Here's how the part is built. I have some questions about the finished solid (model axes, mm). Face numbers are marked on the shaded views. A direction names the side the tool comes from. Round coordinates to 2 decimals unless told otherwise and drop trailing zeros. Write each loop counter-clockwise with the first axis right and the second up, starting at its lowest first coordinate (ties: lowest second). Pieces come first, ordered by that corner, then holes. Notation, with made-up numbers: (10.25, 39.25) - (24.25, 39.25) arc R14 cw to (24.25, 65.25) - close; hole circle Ø2 at (-1.5, 63.25). An arc over 180 degrees is marked (long way). Write item = value, one per line. Start each with the question number.
Item 1: If we section it at A-A (x = 12): Please give me the cut outline in (y, z).
Item 2: If we section it at B-B (y = -110.5): Give the number of separate pieces and of enclosed holes in the cut face, and give its area (3 significant figures).
Item 3: If I drill on line 1 along Z through (x, y) = (9, 0); line 2 along Y through (x, z) = (3.5, -13); line 3 along X through (y, z) = (127, -56.5), over which ranges is the centre line in solid material (lowest first)? Write a range as [from, to].
Item 4: Which directions (+Z, -Z, +X, -X, +Y, -Y) give clear straight access to the entire face, cutting with the end or side of a thin tool? Please do the marked faces 1 and 2.
Item 5: For P1, Ø6, axis at x = 0, y = -110.5, coming from the +Z side; P2, Ø12, axis at y = -100.5, z = 28, coming from the +X side; P3, Ø1.8, axis at x = -1, z = 79, coming from the +Y side, each with a flat end and sliding along its axis, tell me the tip position at first contact or that it passes through.
```python
from build123d import *

# Parameters (mm, degrees)
F0_R          = 150
F0_R_2        = 137.5
F1_DEPTH      = 8
F1_DEPTH_BACK = 8
F0_R_3        = 15
F2_DEPTH      = 3
F2_DEPTH_BACK = 3
F0_R_4        = 11
F3_DEPTH      = 25
F3_DEPTH_BACK = 5
F4_R          = 4


with BuildPart() as f1:
    # F0 (on Right) → F1 (new body, two sides)
    with BuildSketch(Plane.YZ) as f1_sk:
        Circle(F0_R)
        with Locations((2.112069, 0)):
            Circle(F0_R_2, mode=Mode.SUBTRACT)
    extrude(amount=F1_DEPTH)
    extrude(f1_sk.sketch, amount=-F1_DEPTH_BACK)

    # F0 (on Right) → F2 (join, two sides)
    with BuildSketch(Plane.YZ) as f2_sk:
        with Locations((2.112069, 0)):
            Circle(F0_R_2)
        with BuildLine():
            ThreePointArc((-20.96825, -1.5987), (-18.909393, -2.888208), (-17.701314, -4.995877))
            ThreePointArc((-17.701314, -4.995877), (-17.492598, -5.68369), (-17.257166, -6.362822))
            ThreePointArc((-17.257166, -6.362822), (-16.995666, -8.778053), (-17.903363, -11.031452))
            Line((-17.903363, -11.031452), (-80.155489, -96.714153))
            ThreePointArc((-80.155489, -96.714153), (-83.705152, -98.750622), (-87.586694, -97.454111))
            ThreePointArc((-87.586694, -97.454111), (-124.025507, -40.404007), (-127.515568, 27.200141))
            ThreePointArc((-127.515568, 27.200141), (-125.127779, 30.500202), (-121.077051, 30.928621))
            Line((-121.077051, 30.928621), (-20.96825, -1.5987))
        make_face(mode=Mode.SUBTRACT)
        with BuildLine():
            ThreePointArc((67.077994, -115.42357), (0.327024, -132.43861), (-65.941115, -113.6307))
            ThreePointArc((-65.941115, -113.6307), (-68.271016, -110.341527), (-67.417198, -106.402225))
            Line((-67.417198, -106.402225), (-4.959091, -20.436016))
            ThreePointArc((-4.959091, -20.436016), (-3.096475, -18.876406), (-0.718646, -18.378761))
            ThreePointArc((-0.718646, -18.378761), (0, -18.392806), (0.718646, -18.378761))
            ThreePointArc((0.718646, -18.378761), (3.096475, -18.876406), (4.959091, -20.436016))
            Line((4.959091, -20.436016), (68.670621, -108.127414))
            ThreePointArc((68.670621, -108.127414), (69.510512, -112.132647), (67.077994, -115.42357))
        make_face(mode=Mode.SUBTRACT)
        with BuildLine():
            ThreePointArc((131.452799, 28.53327), (127.908721, -41.453278), (89.151697, -99.836241))
            ThreePointArc((89.151697, -99.836241), (85.303528, -101.035698), (81.820873, -99.006358))
            Line((81.820873, -99.006358), (17.903363, -11.031452))
            ThreePointArc((17.903363, -11.031452), (16.995666, -8.778053), (17.257166, -6.362822))
            ThreePointArc((17.257166, -6.362822), (17.492598, -5.68369), (17.701314, -4.995877))
            ThreePointArc((17.701314, -4.995877), (18.909393, -2.888208), (20.96825, -1.5987))
            Line((20.96825, -1.5987), (125.025113, 32.211424))
            ThreePointArc((125.025113, 32.211424), (129.053534, 31.795846), (131.452799, 28.53327))
        make_face(mode=Mode.SUBTRACT)
        with BuildLine():
            ThreePointArc((-119.298215, 52.940673), (-76.904867, 106.299086), (-13.59286, 131.516262))
            ThreePointArc((-13.59286, 131.516262), (-9.680685, 130.290805), (-8, 126.551534))
            Line((-8, 126.551534), (-8, 19.447965))
            ThreePointArc((-8, 19.447965), (-8.590172, 17.091396), (-10.221368, 15.291139))
            ThreePointArc((-10.221368, 15.291139), (-10.81102, 14.880092), (-11.384161, 14.44632))
            ThreePointArc((-11.384161, 14.44632), (-13.600374, 13.451271), (-16.023978, 13.618204))
            Line((-16.023978, 13.618204), (-116.260072, 46.186885))
            ThreePointArc((-116.260072, 46.186885), (-119.274863, 48.890941), (-119.298215, 52.940673))
        make_face(mode=Mode.SUBTRACT)
        Circle(F0_R_3, mode=Mode.SUBTRACT)
        with BuildLine():
            ThreePointArc((13.427143, 131.966439), (78.792322, 107.996809), (122.970872, 54.187837))
            ThreePointArc((122.970872, 54.187837), (122.978837, 50.114524), (119.953547, 47.386968))
            Line((119.953547, 47.386968), (16.023978, 13.618204))
            ThreePointArc((16.023978, 13.618204), (13.600374, 13.451271), (11.384161, 14.44632))
            ThreePointArc((11.384161, 14.44632), (10.81102, 14.880092), (10.221368, 15.291139))
            ThreePointArc((10.221368, 15.291139), (8.590172, 17.091396), (8, 19.447965))
            Line((8, 19.447965), (8, 126.984717))
            ThreePointArc((8, 126.984717), (9.618855, 130.668175), (13.427143, 131.966439))
        make_face(mode=Mode.SUBTRACT)
    extrude(amount=F2_DEPTH)
    extrude(f2_sk.sketch, amount=-F2_DEPTH_BACK)

    # F0 (on Right) → F3 (join, two sides)
    with BuildSketch(Plane.YZ) as f3_sk:
        Circle(F0_R_3)
        Circle(F0_R_4, mode=Mode.SUBTRACT)
    extrude(amount=F3_DEPTH)
    extrude(f3_sk.sketch, amount=-F3_DEPTH_BACK)

    # F4 (on Front) → F5 (revolve, cut)
    with BuildSketch(Plane.XZ):
        with Locations((0, -149.748594)):
            Circle(F4_R)
    revolve(axis=Axis((0, 0, 0), (1, 0, 0)), mode=Mode.SUBTRACT)


solid = f1.part
```
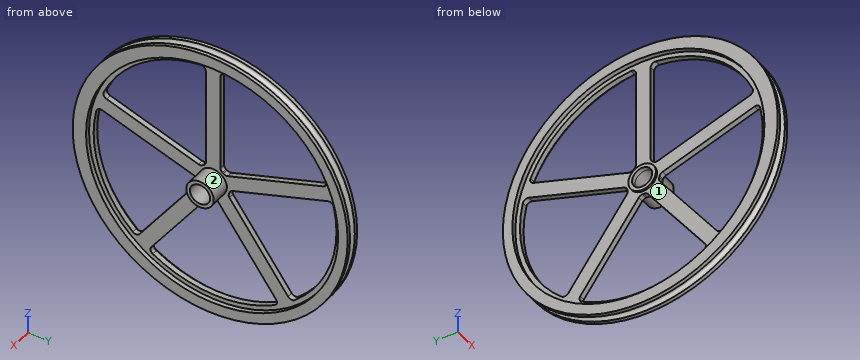
Reply:
q1.outline = circle Ø30 at (0, 0); hole circle Ø22 at (0, 0)
q2.separate_pieces = 3
q2.enclosed_holes = 0
q2.area = 851 mm2
q3.line_1 = [-15, -11], [11, 15]
q3.line_2 = [-147.24, -134.77], [-7.48, 7.48], [139, 147.24]
q3.line_3 = [-3, 3]
q4.face_1 = -X
q4.face_2 = +X
q5.P1 = 98.42
q5.P2 = 3
q5.P3 = 123.31
